The model under review builds one solid part; all positions refer to its coordinate system, in mm. Give positions to 0.01 mm unless a question says otherwise; leave off trailing zeros.
```python
from build123d import *

# Parameters (mm, degrees)
SKETCH_W    = 60
SKETCH_H    = 20
SKETCH_R    = 1.454975
SKETCH_W_2  = 0.08
SKETCH_H_2  = 5
SKETCH_W_3  = 0.085
SKETCH_W_4  = 0.09
SKETCH_W_5  = 0.095
SKETCH_W_6  = 0.1
SKETCH_W_7  = 0.15
SKETCH_W_8  = 0.2
SKETCH_W_9  = 0.25
SKETCH_W_10 = 0.3
SKETCH_W_11 = 0.35
SKETCH_W_12 = 0.4
SKETCH_W_13 = 0.45
SKETCH_W_14 = 0.5
SKETCH_W_15 = 0.55
SKETCH_W_16 = 0.6
SKETCH_W_17 = 0.65
SKETCH_W_18 = 0.7
SKETCH_W_19 = 0.75
SKETCH_W_20 = 0.85
SKETCH_W_21 = 0.9
SKETCH_W_22 = 0.95
SKETCH_W_23 = 1
PAD_DEPTH   = 1


with BuildPart() as part:
    # Sketch → Pad (new body)
    with BuildSketch(Plane.XY):
        with Locations((0, 10)):
            Rectangle(SKETCH_W, SKETCH_H)
        with Locations((-27.249716, 17.255812)):
            Circle(SKETCH_R, mode=Mode.SUBTRACT)
        with Locations((-25.350953, 10)):
            Rectangle(SKETCH_W_2, SKETCH_H_2, mode=Mode.SUBTRACT)
        with Locations((-23.268453, 10)):
            Rectangle(SKETCH_W_3, SKETCH_H_2, mode=Mode.SUBTRACT)
        with Locations((-21.180953, 10)):
            Rectangle(SKETCH_W_4, SKETCH_H_2, mode=Mode.SUBTRACT)
        with Locations((-19.088453, 10)):
            Rectangle(SKETCH_W_5, SKETCH_H_2, mode=Mode.SUBTRACT)
        with Locations((-16.990953, 10)):
            Rectangle(SKETCH_W_6, SKETCH_H_2, mode=Mode.SUBTRACT)
        with Locations((-14.865953, 10)):
            Rectangle(SKETCH_W_7, SKETCH_H_2, mode=Mode.SUBTRACT)
        with Locations((-12.690953, 10)):
            Rectangle(SKETCH_W_8, SKETCH_H_2, mode=Mode.SUBTRACT)
        with Locations((-10.465953, 10)):
            Rectangle(SKETCH_W_9, SKETCH_H_2, mode=Mode.SUBTRACT)
        with Locations((-8.190953, 10)):
            Rectangle(SKETCH_W_10, SKETCH_H_2, mode=Mode.SUBTRACT)
        with Locations((-5.865953, 10)):
            Rectangle(SKETCH_W_11, SKETCH_H_2, mode=Mode.SUBTRACT)
        with Locations((-3.490953, 10)):
            Rectangle(SKETCH_W_12, SKETCH_H_2, mode=Mode.SUBTRACT)
        with Locations((-1.065953, 10)):
            Rectangle(SKETCH_W_13, SKETCH_H_2, mode=Mode.SUBTRACT)
        with Locations((1.409047, 10)):
            Rectangle(SKETCH_W_14, SKETCH_H_2, mode=Mode.SUBTRACT)
        with Locations((3.934047, 10)):
            Rectangle(SKETCH_W_15, SKETCH_H_2, mode=Mode.SUBTRACT)
        with Locations((6.509047, 10)):
            Rectangle(SKETCH_W_16, SKETCH_H_2, mode=Mode.SUBTRACT)
        with Locations((9.134047, 10)):
            Rectangle(SKETCH_W_17, SKETCH_H_2, mode=Mode.SUBTRACT)
        with Locations((11.809047, 10)):
            Rectangle(SKETCH_W_18, SKETCH_H_2, mode=Mode.SUBTRACT)
        with Locations((14.534047, 10)):
            Rectangle(SKETCH_W_19, SKETCH_H_2, mode=Mode.SUBTRACT)
        with Locations((17.334047, 10)):
            Rectangle(SKETCH_W_20, SKETCH_H_2, mode=Mode.SUBTRACT)
        with Locations((20.209047, 10)):
            Rectangle(SKETCH_W_21, SKETCH_H_2, mode=Mode.SUBTRACT)
        with Locations((23.134047, 10)):
            Rectangle(SKETCH_W_22, SKETCH_H_2, mode=Mode.SUBTRACT)
        with Locations((26.109047, 10)):
            Rectangle(SKETCH_W_23, SKETCH_H_2, mode=Mode.SUBTRACT)
    extrude(amount=PAD_DEPTH)


solid = part.part
```
1. To check wall thickness, follow line 1 (Y direction, x = -6, z = 0.8); line 2 (X direction, y = 17, z = 0.6). State the ranges of each line that lie inside material, in increasing order.
2. Take a section at A-A (y = 9.75). Count the separate pieces of the cut face and the enclosed holes in it, and give its area (3 significant figures).
3. Draft analysis for pull direction X (two halves, no side actions). For faces 1 (the flat face through (-0.4, 20, 0.5)), 2 (the flat face through (-12.791, 10, 0.5)), 3 (the flat face through (-8.041, 10, 0.5)), state which applies: pulls with the +X half, pulls with the -X half, needs draft (parallel to the pull), parting line crosses it, or undercut.
Answer:
1. line 1: y = 0 to 7.5, 12.5 to 20
1. line 2: x = -30 to -28.68, -25.82 to 30
2. separate pieces: 23
2. enclosed holes: 0
2. area: 50.0 mm2
3. face 1: needs draft
3. face 2: undercut
3. face 3: undercut
